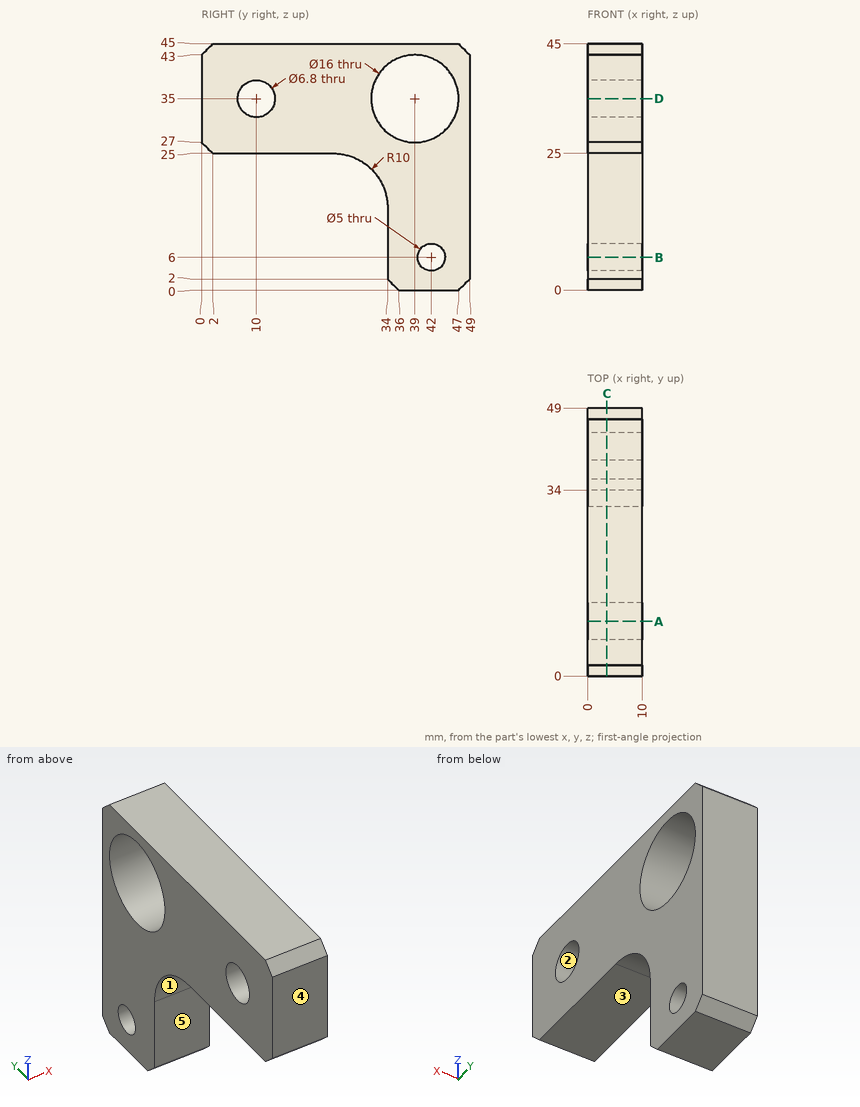
Design review of the part shown in the three views and the two pictorial views. Dimensions are in mm from the part's minimum x, y and z. A direction names the side the tool comes from. Round coordinates to 2 decimals unless told otherwise and drop trailing zeros. Order: outer loops, then holes, each group sorted by start corner. A loop starts at its lowest first (then second) coordinate and runs counter-clockwise, first axis right, second up. Notation, with made-up numbers: (10.5, -10) - (53.5, -10) arc R32 cw to (53.5, 29) - close; hole circle Ø1 at (86.25, -10). An arc over 180 degrees is marked (long way). Answer in a Markdown table with one row per item.
(1) Take a section at B-B on z = 6. Write out the cut boundary in (x, y), plus the area to 3 significant figures.
Result set:
| item | result |
|---|---|
| outline | (0, 34) - (10, 34) - (10, 39.5) - (0, 39.5) - close; (0, 44.5) - (10, 44.5) - (10, 49) - (0, 49) - close |
| area | 100 mm2 |
(2) Take a section at A-A on y = 10. Write out the cut boundary in (x, z), plus the area to 3 significant figures.
Result set:
| item | result |
|---|---|
| outline | (0, 25) - (10, 25) - (10, 31.6) - (0, 31.6) - close; (0, 38.4) - (10, 38.4) - (10, 45) - (0, 45) - close |
| area | 132 mm2 |
(3) Take a section at C-C on x = 3.5. Write out the cut boundary in (y, z).
Result set:
| item | result |
|---|---|
| outline | (0, 27) - (2, 25) - (24, 25) arc R10 cw to (34, 15) - (34, 2) - (36, 0) - (47, 0) - (49, 2) - (49, 43) - (47, 45) - (2, 45) - (0, 43) - close; hole circle Ø6.8 at (10, 35); hole circle Ø16 at (39, 35); hole circle Ø5 at (42, 6) |
(4) Clearance check with flat-ended pins moving along their axes: P1, Ø8, axis at y = 22, z = 22, coming from the -X side; P2, Ø3, axis at x = 6.5, y = 8.5, coming from the -Z side. State where each tip first meets the part, or that it passes through.
Result set:
| item | result |
|---|---|
| P1 | stops at x = 0 |
| P2 | stops at z = 25 |
(5) Take a section at D-D on z = 35. Write out the cut boundary in (x, y).
Result set:
| item | result |
|---|---|
| outline | (0, 0) - (10, 0) - (10, 6.6) - (0, 6.6) - close; (0, 13.4) - (10, 13.4) - (10, 31) - (0, 31) - close; (0, 47) - (10, 47) - (10, 49) - (0, 49) - close |
(6) For line 1 (Y direction, x = 3, z = 35); line 2 (Z direction, x = 4, y = 41); line 3 (Y direction, x = 5.5, z = 36.5), list the stretches that pass through material, from the lowest coordinate up. Write a range as from..to.
Result set:
| item | result |
|---|---|
| line 1 | y = 0..6.6, 13.4..31, 47..49 |
| line 2 | z = 0..3.71, 8.29..27.25, 42.75..45 |
| line 3 | y = 0..6.95, 13.05..31.14, 46.86..49 |
(7) Mouldability with a two-part tool opening along Y and no side actions: class the marked faces 1, 2 and 3 as released by +Y, released by -Y, zero draft, split by the parting line, or undercut.
Result set:
| item | result |
|---|---|
| face 1 | released by -Y |
| face 2 | undercut |
| face 3 | zero draft |
(8) Machinability: for the marked faces 4 and 5, which of the approach directions +Z, -Z, +X, -X, +Y, -Y give a long, thin tool a straight path to every point of the face, cutting with its end or side? Answer none if there is none.
Result set:
| item | result |
|---|---|
| face 4 | +Z, -Z, +X, -X, -Y |
| face 5 | -Z, +X, -X, -Y |
